Input: dimensioned drawing with shaded views. Units: mm. Origin: part minimum x, y, z. A direction names the side the tool comes from. Round coordinates to 2 decimals unless told otherwise and drop trailing zeros. Order: outer loops, then holes, each group sorted by start corner. A loop starts at its lowest first (then second) coordinate and runs counter-clockwise, first axis right, second up. Notation, with made-up numbers: M 17.25,85.25 L 48.25,85.25 A28 ccw 48.25,107.25 Z; hole C -15,75 d3. An arc over 180 degrees is marked long. One line per question, with ' | ' between items.
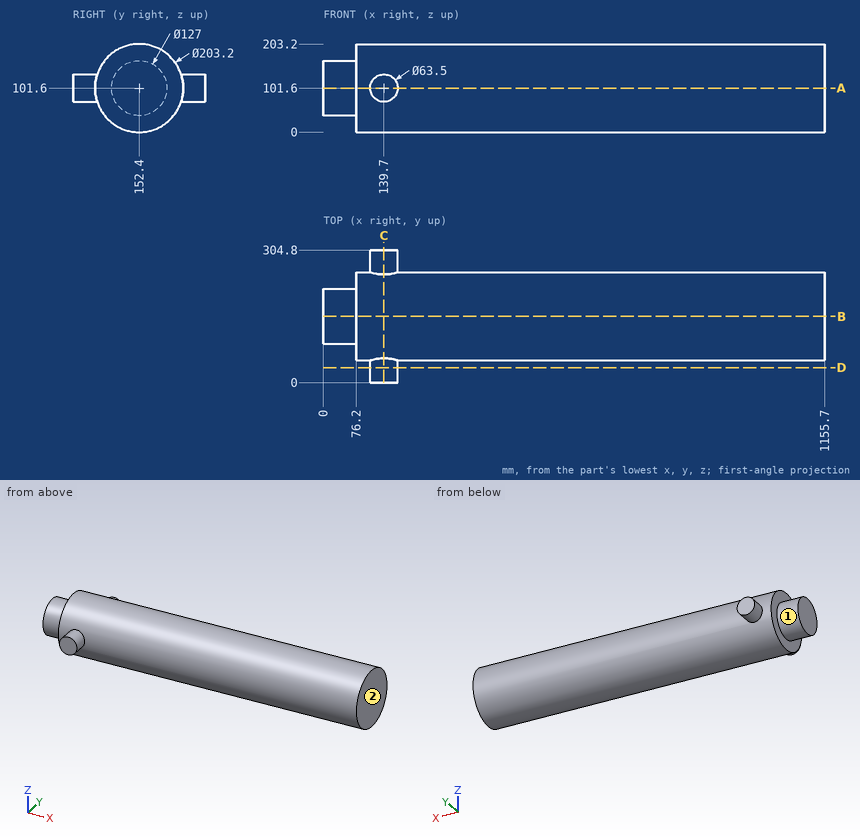
Item 1: Access query for the marked faces 1 and 2. Directions: +Z, -Z, +X, -X, +Y, -Y. A direction counts if a zero-diameter tool reaches every point of the face in a straight line with its end or side. Return the directions, or none.
Report:
face 1: -X | face 2: +Z, -Z, +X, +Y, -Y
Item 2: Section query A-A, the plane z = 101.6. Return loops of the section in (x, y).
Report:
outline: M 0,88.9 L 76.2,88.9 L 76.2,50.8 L 107.95,50.8 L 107.95,0 L 171.45,0 L 171.45,50.8 L 1155.7,50.8 L 1155.7,254 L 171.45,254 L 171.45,304.8 L 107.95,304.8 L 107.95,254 L 76.2,254 L 76.2,215.9 L 0,215.9 Z
Item 3: Section query C-C, the plane x = 139.7. Return loops of the section in (y, z), plus the area to 3 significant figures.
Report:
outline: M 0,69.85 L 55.89,69.85 A101.6 ccw 248.91,69.85 L 304.8,69.85 L 304.8,133.35 L 248.91,133.35 A101.6 ccw 55.89,133.35 L 0,133.35 Z | area: 39,100 mm²
Item 4: Section query D-D, the plane y = 34.5. Return loops of the section in (x, z), plus the area to 3 significant figures.
Report:
outline: C 139.7,101.6 d63.5 | area: 3,170 mm²
Item 5: First-contact query: pin 1 (1.5 mm diameter, centred on x = 223, z = 37, fed in from +Y); pin 2 (2 mm diameter, centred on x = 326.5, z = 147.5, fed in from -Y); pin 3 (10 mm diameter, centred on x = 871, y = 233, fed in from -Z); pin 4 (1 mm diameter, centred on y = 110, z = 81.5, fed in from -X). Flat tips, straight axial feed; report the tip coordinate or a pass-through.
Report:
pin 1: y = 231.43 | pin 2: y = 61.26 | pin 3: z = 33.72 | pin 4: x = 0
Item 6: Section query B-B, the plane y = 152.4. Return loops of the section in (x, z), plus the area to 3 significant figures.
Report:
outline: M 0,38.1 L 76.2,38.1 L 76.2,0 L 1155.7,0 L 1155.7,203.2 L 76.2,203.2 L 76.2,165.1 L 0,165.1 Z | area: 229,000 mm²
Item 7: Line query: line 1 along Y through (x, z) = (354, 98); line 2 along X through (y, z) = (97, 152); line 3 along Z through (x, y) = (221, 158). Output: solid intervals per line, ascending. Write a range as from..to.
Report:
line 1: 50.86..253.94 | line 2: 76.2..1155.7 | line 3: 0.15..203.05
